Part model, mm, in its own coordinate system. A direction names the side the tool comes from. Round coordinates to 2 decimals unless told otherwise and drop trailing zeros. Write each loop counter-clockwise with the first axis right and the second up, starting at its lowest first coordinate (ties: lowest second). Pieces come first, ordered by that corner, then holes.
from build123d import *

# Parameters (mm, degrees)
F1_DEPTH  = 12.7
F2_W      = 12.7
F2_H      = 12.7
F3_DEPTH  = 12.7
F4_W      = 5.08
F4_H      = 10.16
F6_DEPTH  = 12.7
F7_W      = 10.16
F7_H      = 5.08
F8_DEPTH  = 12.7
F9_W      = 5.08
F9_H      = 10.16
F10_DEPTH = 12.7
F11_W     = 10.16
F11_H     = 10.16
F12_DEPTH = 12.7


with BuildPart() as f1:
    # F0 (on Top) → F1 (new body)
    with BuildSketch(Plane.XY):
        Polygon((0, 12.7), (0, 0), (38.1, 0), (38.1, 12.7), (25.4, 12.7), (25.4, 25.4), (12.7, 25.4), (12.7, 12.7), align=None)
    extrude(amount=F1_DEPTH)

    # F2 (on face) → F3 (join)
    with BuildSketch(Plane.XY.offset(12.7)):
        with Locations((19.05, 6.35)):
            Rectangle(F2_W, F2_H)
    extrude(amount=F3_DEPTH)

    # F4 (on face) → F6 (cut)
    with BuildSketch(Plane.YZ.offset(38.1)):
        with Locations((3.81, 6.35)):
            Rectangle(F4_W, F4_H)
        with BuildLine():
            Line((6.35, 11.43), (6.35, 1.27))
            ThreePointArc((6.35, 1.27), (11.43, 6.35), (6.35, 11.43))
        make_face()
    extrude(amount=-F6_DEPTH, mode=Mode.SUBTRACT)

    # F7 (on face) → F8 (cut)
    with BuildSketch(Plane.XY.offset(25.4)):
        with Locations((19.05, 3.81)):
            Rectangle(F7_W, F7_H)
        with BuildLine():
            Line((13.97, 6.35), (24.13, 6.35))
            ThreePointArc((24.13, 6.35), (19.05, 11.43), (13.97, 6.35))
        make_face()
    extrude(amount=-F8_DEPTH, mode=Mode.SUBTRACT)

    # F9 (on face) → F10 (cut)
    with BuildSketch(Plane(origin=(0, 0, 0), x_dir=(0, -1, 0), z_dir=(-1, 0, 0))):
        with Locations((-3.81, 6.35)):
            Rectangle(F9_W, F9_H)
        with BuildLine():
            Line((-6.35, 1.27), (-6.35, 11.43))
            ThreePointArc((-6.35, 11.43), (-11.43, 6.35), (-6.35, 1.27))
        make_face()
    extrude(amount=-F10_DEPTH, mode=Mode.SUBTRACT)

    # F11 (on face) → F12 (cut)
    with BuildSketch(Plane(origin=(0, 25.4, 0), x_dir=(-1, 0, 0), z_dir=(0, 1, 0))):
        with Locations((-19.05, 6.35)):
            Rectangle(F11_W, F11_H)
    extrude(amount=-F12_DEPTH, mode=Mode.SUBTRACT)


solid = f1.part
Q1. Saw through at C-C, the plane y = 12. Write the cut outline in (x, z), and give its area (3 significant figures).
Q2. Saw through at A-A, the plane z = 20.5. Write the cut outline in (x, y), and give its area (3 significant figures).
Q3. Tool access for faces 1 (the cylindrical face through (6.26, 11.43, 6.46)), 2 (the flat face through (25.4, 6, 19)), 3 (the flat face through (6, 6, 12.7)), 4 (the flat face through (19, 12.7, 6)), 5 (the flat face through (24.13, 4, 19)): list every direction of +Z, -Z, +X, -X, +Y, -Y with a clear straight run to the whole face (end or side of a thin tool).
Q4. Wall check: line 1 (X direction, y = 3.5, z = 18.75); line 2 (Z direction, x = 8.5, y = 6.25). Give the ranges that are in metal, low to high.
Q5. Saw through at B-B, the plane y = 21.25. Write the cut outline in (x, z), and give its area (3 significant figures).
Q6. Drop flat-ended pins along their axis: P1, Ø2.5, axis at y = 2.5, z = 20.5, coming from the +X side; P2, Ø3, axis at x = 32.5, z = 6, coming from the +Y side; P3, Ø4, axis at x = 30.5, y = 4, coming from the +Z side. Give the stop position or say it passes through.
Q7. Two-plate mould, pull along X, no slides. Class faces 6 (the flat face through (0, 11, 3)), 7 (the flat face through (32, 12.7, 6)), 8 (the flat face through (19, 19, 11.43)): released by +X, released by -X, zero draft, split by the parting line, or undercut.
Q8. Saw through at D-D, the plane x = 19.05. Write the cut outline in (y, z), and give its area (3 significant figures).
Computed:
1. outline: (0, 0) - (38.1, 0) - (38.1, 12.7) - (25.4, 12.7) - (25.4, 25.4) - (12.7, 25.4) - (12.7, 12.7) - (0, 12.7) - close
1. area: 645 mm2
2. outline: (12.7, 0) - (25.4, 0) - (25.4, 12.7) - (12.7, 12.7) - close; hole (13.97, 1.27) - (24.13, 1.27) - (24.13, 6.35) arc R5.08 ccw to (13.97, 6.35) - close
2. area: 69.1 mm2
3. face 1: -X
3. face 2: +Z, +X, +Y, -Y
3. face 3: +Z, -X, +Y, -Y
3. face 4: +Y
3. face 5: +Z
4. line 1: x = 12.7 to 13.97, 24.13 to 25.4
4. line 2: z = 0 to 1.27, 11.43 to 12.7
5. outline: (12.7, 0) - (25.4, 0) - (25.4, 12.7) - (12.7, 12.7) - close; hole (13.97, 1.27) - (24.13, 1.27) - (24.13, 11.43) - (13.97, 11.43) - close
5. area: 58.1 mm2
6. P1: stops at x = 25.4
6. P2: stops at y = 12.7
6. P3: stops at z = 12.7
7. face 6: released by -X
7. face 7: zero draft
7. face 8: undercut
8. outline: (0, 0) - (25.4, 0) - (25.4, 1.27) - (12.7, 1.27) - (12.7, 11.43) - (25.4, 11.43) - (25.4, 12.7) - (12.7, 12.7) - (12.7, 25.4) - (11.43, 25.4) - (11.43, 12.7) - (1.27, 12.7) - (1.27, 25.4) - (0, 25.4) - close
8. area: 226 mm2
